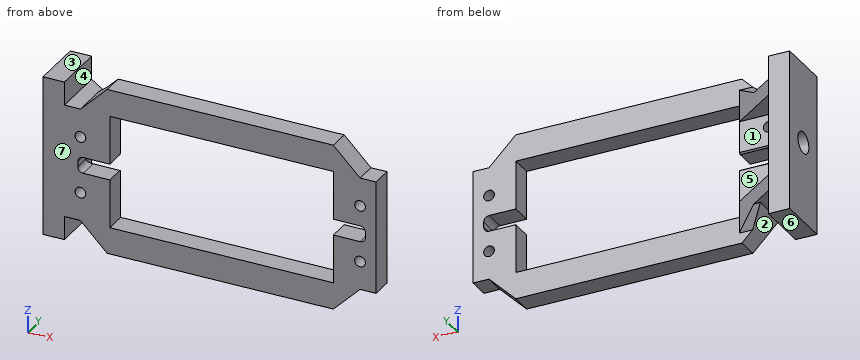
from build123d import *

# Parameters (mm, degrees)
SKETCH1_R           = 1
BOSS_EXTRUDE1_DEPTH = 4
FILLET1_R           = 1
SKETCH2_W           = 30
SKETCH2_H           = 10
BOSS_EXTRUDE2_DEPTH = 4
SKETCH3_W           = 8.5
SKETCH3_H           = 3
BOSS_EXTRUDE3_DEPTH = 6
CUT_EXTRUDE1_DEPTH  = 44.611924975
CHAMFER3_SIZE       = 3
CUT_EXTRUDE2_REACH  = 66.997
SKETCH5_R           = 2


with BuildPart() as part:
    # Sketch1 → Boss-Extrude1 (new body)
    with BuildSketch(Plane(origin=(0, 0, 0), x_dir=(1, 0, 0), z_dir=(0, 1, 0))):
        Polygon((-21.4, 15.6), (-26.4, 10.6), (-29.4, 10.6), (-29.4, -10.6), (-26.4, -10.6), (-21.4, -15.6), (20.9, -15.6), (25.9, -10.6), (28.9, -10.6), (28.9, 10.6), (25.9, 10.6), (20.9, 15.6), align=None)
        Polygon((20.9, -1.5), (20.9, -10.6), (-20.9, -10.6), (-20.9, -1.5), (-26.9, -1.5), (-26.9, 1.5), (-20.9, 1.5), (-20.9, 10.6), (20.9, 10.6), (20.9, 1.5), (26.9, 1.5), (26.9, -1.5), align=None, mode=Mode.SUBTRACT)
        with Locations(Location((-26.4, 5.3, 0), (0, 0, 270))):
            Circle(SKETCH1_R, mode=Mode.SUBTRACT)
        with Locations(Location((-26.4, -5.3, 0), (0, 0, 270))):
            Circle(SKETCH1_R, mode=Mode.SUBTRACT)
        with Locations(Location((25.9, -5.3, 0), (0, 0, 270))):
            Circle(SKETCH1_R, mode=Mode.SUBTRACT)
        with Locations(Location((25.9, 5.3, 0), (0, 0, 270))):
            Circle(SKETCH1_R, mode=Mode.SUBTRACT)
    extrude(amount=BOSS_EXTRUDE1_DEPTH)

    # Fillet1
    fillet1_edges = [part.edges().sort_by_distance(p)[0] for p in [
        (26.9, 2, 1.5),
        (26.9, 2, -1.5),
        (-26.9, 2, -1.5),
        (-26.9, 2, 1.5),
    ]]
    fillet(fillet1_edges, radius=FILLET1_R)

    # Sketch2 → Boss-Extrude2 (add)
    with BuildSketch(Plane.ZY.offset(29.4)):
        with Locations((0, 5)):
            Rectangle(SKETCH2_W, SKETCH2_H)
    extrude(amount=BOSS_EXTRUDE2_DEPTH)

    # Sketch3 → Boss-Extrude3 (add)
    with BuildSketch(Plane(origin=(0, 4, 0), x_dir=(1, 0, 0), z_dir=(0, 1, 0))):
        with Locations((-25.15, -9.1)):
            Rectangle(SKETCH3_W, SKETCH3_H)
        with Locations((-25.15, 9.1)):
            Rectangle(SKETCH3_W, SKETCH3_H)
    extrude(amount=BOSS_EXTRUDE3_DEPTH)

    # Sketch4 → Cut-Extrude1 (cut, through all)
    with BuildSketch(Plane(origin=(0, 0, -10.6), x_dir=(-1, 0, 0), z_dir=(0, 0, -1))):
        Polygon((20.9, 4), (29.4, 10), (20.9, 10), align=None)
    extrude(amount=-CUT_EXTRUDE1_DEPTH, mode=Mode.SUBTRACT)

    # Chamfer3
    # the kernel refuses this chamfer: 3 mm, written as the material it adds along each edge
    with BuildSketch(Plane(origin=(-13.184951036, 4, 10.6), x_dir=(0, -0.02749587661058635, 0.9996219169112968), z_dir=(-1, 0, 0))) as chamfer3_piece_1_section:
        Polygon((CHAMFER3_SIZE * 0.999621916911, CHAMFER3_SIZE * 0.0274958766106), (-CHAMFER3_SIZE * 0.0274958766106, CHAMFER3_SIZE * 0.999621916911), (0, 0), align=None)
    chamfer3_piece_1 = extrude(amount=20.930097928, mode=Mode.PRIVATE)
    chamfer3_piece_1 = split(chamfer3_piece_1, bisect_by=Plane(origin=(-24.611993243, 4.851351351, 12.388006757), z_dir=(0.7071067811865483, 0, -0.7071067811865467)), keep=Keep.TOP, mode=Mode.PRIVATE)
    chamfer3_piece_1 = split(chamfer3_piece_1, bisect_by=Plane(origin=(-23.221105892, 5.638427689, 11.552702703), z_dir=(-0.5766831975986547, -0.8169678632647621, 0)), keep=Keep.TOP, mode=Mode.PRIVATE)
    add(chamfer3_piece_1)
    with BuildSketch(Plane(origin=(-13.184951036, 4, -10.6), x_dir=(-1.6712331566303747e-15, -0.02749587661058635, -0.9996219169112968), z_dir=(-1, 0, 0))) as chamfer3_piece_2_section:
        Polygon((CHAMFER3_SIZE * 0.999621916911, -CHAMFER3_SIZE * 0.0274958766106), (-CHAMFER3_SIZE * 0.0274958766106, -CHAMFER3_SIZE * 0.999621916911), (0, 0), align=None)
    chamfer3_piece_2 = extrude(amount=20.930097928, mode=Mode.PRIVATE)
    chamfer3_piece_2 = split(chamfer3_piece_2, bisect_by=Plane(origin=(-24.611993243, 4.851351351, -12.388006757), z_dir=(0.7071067811865487, 0, 0.7071067811865465)), keep=Keep.TOP, mode=Mode.PRIVATE)
    chamfer3_piece_2 = split(chamfer3_piece_2, bisect_by=Plane(origin=(-23.221105892, 5.638427689, -11.552702703), z_dir=(-0.5766831975986547, -0.8169678632647621, 0)), keep=Keep.TOP, mode=Mode.PRIVATE)
    add(chamfer3_piece_2)

    # Sketch5 → Cut-Extrude2 (cut, up to next)
    with BuildSketch(Plane.ZY.offset(33.4), mode=Mode.PRIVATE) as cut_extrude2_sk1:
        with Locations((0, 5)):
            Circle(SKETCH5_R)
    cut_extrude2_tool1 = extrude(cut_extrude2_sk1.sketch, amount=-CUT_EXTRUDE2_REACH, mode=Mode.PRIVATE) & part.part
    add(cut_extrude2_tool1.solids().sort_by_distance((-33.4, 5, 0))[0], mode=Mode.SUBTRACT)


solid = part.part
Work out the finished part from the listing and answer in its coordinate system (mm). Face numbers are marked on the shaded views. A direction names the side the tool comes from. Give positions to 0.01 mm unless a question says otherwise; leave off trailing zeros. Loops run counter-clockwise (first coordinate to the right, second up) from the corner with the lowest first, then second, coordinate; pieces in that order, holes last. Notation, with made-up numbers: (54, 9) -> (95, 9) arc R18 cw to (95, 18) -> close; hole circle Ø8 at (81.5, 59.5). An arc over 180 degrees is marked (long way). Use a Markdown table: item, result. Add a question column.
1. Find the intervals of material crossed by probe 1 along X at (y, z) = (1, -5.3); probe 2 along Z at (x, y) = (-14, 3.75); probe 3 along X at (y, z) = (1.5, 7), in increasing order.
2. Section D-D on z = 9 is taken. Determine the outline of the cut face in (x, y).
3. For the marked faces 1, 2, 3 and 4, determine the directions among +Z, -Z, +X, -X, +Y, -Y from which every point of the face is accessible in a straight line to the end or side of a thin tool.
4. Section A-A on x = 22 is taken. Determine the outline of the cut face in (y, z), and give its area (3 significant figures).
5. Section B-B on z = -7 is taken. Determine the outline of the cut face in (x, y).
6. Section C-C on y = 5.75 is taken. Determine the outline of the cut face in (x, z), and give its area (3 significant figures).
7. Flat-ended cylindrical pins translate along their axes: pin 1 Ø2.5 at (x, y) = (27.5, 1) entering from +Z; pin 2 Ø1.8 at (x, y) = (-26.5, 7) entering from -Z; pin 3 Ø3.5 at (y, z) = (6, -13.5) entering from +X. Find the tip coordinate at first contact, or state that the pin passes through.
8. Determine the mould class of the marked faces 5, 6 and 7 for opening direction Z: released by +Z, released by -Z, zero draft, split by the parting line, or undercut.
Results below:
| question | item | result |
|---|---|---|
| 1 | probe 1 | x = -33.4 to -27.4, -25.4 to -20.9, 20.9 to 24.9, 26.9 to 28.9 |
| 1 | probe 2 | z = -15.6 to -10.6, 10.6 to 15.6 |
| 1 | probe 3 | x = -33.4 to -20.9, 20.9 to 28.9 |
| 2 | outline | (-33.4, 0) -> (-20.9, 0) -> (-20.9, 4) -> (-29.4, 10) -> (-33.4, 10) -> close; (20.9, 0) -> (28.9, 0) -> (28.9, 4) -> (20.9, 4) -> close |
| 3 | face 1 | +X, +Y |
| 3 | face 2 | -Z, +Y, -Y |
| 3 | face 3 | +Z, -X, +Y, -Y |
| 3 | face 4 | +Z, +Y, -Y |
| 4 | outline | (0, -14.5) -> (4, -14.5) -> (4, -1.5) -> (0, -1.5) -> close; (0, 1.5) -> (4, 1.5) -> (4, 14.5) -> (0, 14.5) -> close |
| 4 | area | 104 mm^2 |
| 5 | outline | (-33.4, 0) -> (-20.9, 0) -> (-20.9, 4) -> (-29.4, 4) -> (-29.4, 10) -> (-33.4, 10) -> close; (20.9, 0) -> (28.9, 0) -> (28.9, 4) -> (20.9, 4) -> close |
| 6 | outline | (-33.4, -15) -> (-29.4, -15) -> (-29.4, -10.6) -> (-26.4, -10.6) -> (-25.15, -11.85) -> (-23.38, -11.85) -> (-23.38, -7.6) -> (-29.4, -7.6) -> (-29.4, -1.85) -> (-33.4, -1.85) -> close; (-33.4, 1.85) -> (-29.4, 1.85) -> (-29.4, 7.6) -> (-23.38, 7.6) -> (-23.38, 11.85) -> (-25.15, 11.85) -> (-26.4, 10.6) -> (-29.4, 10.6) -> (-29.4, 15) -> (-33.4, 15) -> close |
| 6 | area | 147 mm^2 |
| 7 | pin 1 | stops at z = 10.6 |
| 7 | pin 2 | stops at z = -11.18 |
| 7 | pin 3 | stops at x = -21.26 |
| 8 | face 5 | undercut |
| 8 | face 6 | released by -Z |
| 8 | face 7 | zero draft |
